from build123d import *

# Parameters (mm, degrees)
SKETCH1_R           = 13
SKETCH1_R_2         = 4.95
BOSS_EXTRUDE1_DEPTH = 29.6
SKETCH2_R           = 4.95
BOSS_EXTRUDE3_DEPTH = 8.650573
SKETCH3_R           = 4.95
SKETCH3_R_2         = 3.9
BOSS_EXTRUDE4_DEPTH = 11.85


with BuildPart() as part:
    # Sketch1 → Boss-Extrude1 (new body)
    with BuildSketch(Plane(origin=(0, 0, 0), x_dir=(1, 0, 0), z_dir=(0, 1, 0))):
        Circle(SKETCH1_R)
        Circle(SKETCH1_R_2, mode=Mode.SUBTRACT)
    extrude(amount=BOSS_EXTRUDE1_DEPTH)

    # Sketch2 → Boss-Extrude3 (add)
    with BuildSketch(Plane(origin=(0, 18.650573, 0), x_dir=(1, 0, 0), z_dir=(0, 1, 0))):
        Circle(SKETCH2_R)
    extrude(amount=-BOSS_EXTRUDE3_DEPTH)

    # Sketch3 → Boss-Extrude4 (add)
    with BuildSketch(Plane.XZ):
        Circle(SKETCH3_R)
        Circle(SKETCH3_R_2, mode=Mode.SUBTRACT)
    extrude(amount=-BOSS_EXTRUDE4_DEPTH)


solid = part.part
Geometry check sheet. Reference: the model listing, model coordinates, mm. A direction names the side the tool comes from. Coordinates: 2 decimals unless noted, no trailing zeros. Write each loop counter-clockwise with the first axis right and the second up, starting at its lowest first coordinate (ties: lowest second). Pieces come first, ordered by that corner, then holes. Notation, with made-up numbers: (35, 64) -> (91, 64) arc R25 cw to (91, 99) -> close; hole circle Ø3 at (21, 71). An arc over 180 degrees is marked (long way). One line per question, with ' | ' between items.
1. Cross-section at D-D on y = 11. Record the cut outline in (x, z), and give its area (3 significant figures).
Answers:
outline: circle Ø26 at (0, 0) | area: 531 mm²
2. Cross-section at C-C on z = 0. Record the cut outline in (x, y), and give its area (3 significant figures).
Answers:
outline: (-13, 0) -> (-3.9, 0) -> (-3.9, 10) -> (3.9, 10) -> (3.9, 0) -> (13, 0) -> (13, 29.6) -> (4.95, 29.6) -> (4.95, 18.65) -> (-4.95, 18.65) -> (-4.95, 29.6) -> (-13, 29.6) -> close | area: 583 mm²
3. Set-up check for faces 1 (the flat face through (0, 18.651, 0)), 2 (the cylindrical face through (-2.87, 4.93, 2.64)), 3 (the flat face through (6, 29.6, 0)): record each of +Z, -Z, +X, -X, +Y, -Y from which the full face is reachable in a straight line by a thin tool's end or side.
Answers:
face 1: +Y | face 2: -Y | face 3: +Z, -Z, +X, -X, +Y
4. Cross-section at B-B on y = 27. Record the cut outline in (x, z), and give its area (3 significant figures).
Answers:
outline: circle Ø26 at (0, 0); hole circle Ø9.9 at (0, 0) | area: 454 mm²
5. Cross-section at A-A on x = 0. Record the cut outline in (y, z), and give its area (3 significant figures).
Answers:
outline: (0, -13) -> (29.6, -13) -> (29.6, -4.95) -> (18.65, -4.95) -> (18.65, 4.95) -> (29.6, 4.95) -> (29.6, 13) -> (0, 13) -> (0, 3.9) -> (10, 3.9) -> (10, -3.9) -> (0, -3.9) -> close | area: 583 mm²
6. Draft check along Z on faces 4 (the cylindrical face through (4.72, 24.05, -1.49)), 5 (the flat face through (3, 0, 3)), 6 (the cylindrical face through (-10.316, 14.593, 7.91)). Enter one of: +Z half, -Z half, draft (parallel to the pull), parting line (faces both ways), or undercut.
Answers:
face 4: undercut | face 5: draft | face 6: parting line
7. Thickness scan on probe 1 along Z at (x, y) = (0, 3.5); probe 2 along Z at (x, y) = (0, 25.25). Record the ranges inside material, lowest first. Write a range as from..to.
Answers:
probe 1: z = -13..-3.9, 3.9..13 | probe 2: z = -13..-4.95, 4.95..13
8. Depth check by flat-ended pin: pin 1 Ø6 at (x, z) = (0, 0) entering from -Y; pin 2 Ø4 at (y, z) = (3.5, 5.5) entering from +X; pin 3 Ø5 at (x, y) = (7, 12) entering from -Z. Enter the tip coordinate at first touch or a pass-through.
Answers:
pin 1: stops at y = 10 | pin 2: stops at x = 12.52 | pin 3: stops at z = -12.2
